```python
from build123d import *

# Parameters (mm, degrees)
BASE_FLANGE1_DEPTH                            = 43.6626
SKETCH3_W                                     = 39.3553177
SKETCH3_H                                     = 59.329005091
CUT_EXTRUDE1_DEPTH                            = 221.446361168
CSK_FOR_8_FLAT_HEAD_MACHINE_SCREW1_AT_2_COUNT = 2
CSK_FOR_8_FLAT_HEAD_MACHINE_SCREW1_AT_2_PITCH = 34.9504
SKETCH6_R                                     = 3.175
SKETCH6_R_2                                   = 2.0193
SKETCH6_R_3                                   = 2.7051
CUT_EXTRUDE2_DEPTH                            = 7.62
CUT_EXTRUDE3_REACH                            = 258.55
SKETCH7_R                                     = 2.7051
CE_00_NOTCH_FOR_WIRE_REACH                    = 222.446


# Sheet-metal steps are written as plain solids
with BuildPart() as part:
    # Sketch1 → Base-Flange1 (new, symmetric)
    with BuildSketch(Plane.XY):
        with BuildLine():
            Line((139.7, -25.4), (139.7, -40.559570335))
            ThreePointArc((139.7, -40.559570335), (139.568524729, -41.220541159), (139.194114832, -41.780885168))
            Line((139.194114832, -41.780885168), (-50.802114832, -231.777114832))
            ThreePointArc((-50.802114832, -231.777114832), (-51.362458841, -232.151524729), (-52.023429665, -232.283))
            Line((-52.023429665, -232.283), (-70.358, -232.283))
            Line((-70.358, -232.283), (-70.358, -234.569))
            Line((-70.358, -234.569), (-52.023429665, -234.569))
            ThreePointArc((-52.023429665, -234.569), (-50.487644514, -234.26351334), (-49.185668731, -233.393560934))
            Line((-49.185668731, -233.393560934), (140.810560934, -43.397331269))
            ThreePointArc((140.810560934, -43.397331269), (141.68051334, -42.095355486), (141.986, -40.559570335))
            Line((141.986, -40.559570335), (141.986, -25.4))
            Line((141.986, -25.4), (139.7, -25.4))
        make_face()
    extrude(amount=BASE_FLANGE1_DEPTH, both=True)

    # Sketch3 → Cut-Extrude1 (cut, through all)
    with BuildSketch(Plane(origin=(92.103946102, -92.103946102, 0), x_dir=(0, 0, -1), z_dir=(0.7071067811865464, -0.7071067811865487, 0))):
        with Locations((-56.20285885, -229.689502546)):
            Rectangle(SKETCH3_W, SKETCH3_H)
        with Locations((56.20285885, -229.689502546)):
            Rectangle(SKETCH3_W, SKETCH3_H)
    extrude(amount=-CUT_EXTRUDE1_DEPTH, mode=Mode.SUBTRACT)

    # Sketch4 → CSK for #8 Flat Head Machine Screw1 (revolve, cut)
    with BuildSketch(Plane(origin=(141.986, -33.3502, -17.4752), x_dir=(0, 0, -1), z_dir=(0, 1, 0))):
        Polygon((0, 0), (0, 2.286), (2.7051, 2.286), (2.7051, 1.738551774), (4.2164, 0), align=None)
    csk_for_8_flat_head_machine_screw1 = revolve(axis=Axis((148.336, -33.3502, -17.4752), (-1, 0, 0)), mode=Mode.SUBTRACT)

    # CSK for #8 Flat Head Machine Screw1 at 2: CSK for #8 Flat Head Machine Screw1 ×2
    with Locations(*[(0, 0, i * CSK_FOR_8_FLAT_HEAD_MACHINE_SCREW1_AT_2_PITCH) for i in range(1, CSK_FOR_8_FLAT_HEAD_MACHINE_SCREW1_AT_2_COUNT)]):
        add(csk_for_8_flat_head_machine_screw1, mode=Mode.SUBTRACT)

    # Sketch6 → Cut-Extrude2 (cut)
    with BuildSketch(Plane(origin=(92.103946102, -92.103946102, 0), x_dir=(0, 0, -1), z_dir=(0.7071067811865465, -0.7071067811865486, 0))):
        with Locations(Location((0, 56.896984938, 0), (0, 0, 90))):
            Circle(SKETCH6_R)
        with Locations(Location((25.4, 44.196984938, 0), (0, 0, 90))):
            Circle(SKETCH6_R_2)
        with Locations(Location((25.4, -32.003015062, 0), (0, 0, 90))):
            Circle(SKETCH6_R_2)
        with Locations(Location((25.4, -108.203015062, 0), (0, 0, 90))):
            Circle(SKETCH6_R_2)
        with Locations(Location((-25.4, -108.203015062, 0), (0, 0, 90))):
            Circle(SKETCH6_R_2)
        with Locations(Location((-25.4, -32.003015062, 0), (0, 0, 90))):
            Circle(SKETCH6_R_2)
        with Locations(Location((-25.4, 44.196984938, 0), (0, 0, 90))):
            Circle(SKETCH6_R_2)
        with Locations(Location((0, -32.003015062, 0), (0, 0, 90))):
            Circle(SKETCH6_R_3)
        with Locations(Location((25.4, -184.403015062, 0), (0, 0, 90))):
            Circle(SKETCH6_R_2)
        with Locations(Location((-25.4, -184.403015062, 0), (0, 0, 90))):
            Circle(SKETCH6_R_2)
        with Locations(Location((0, -83.518444727, 0), (0, 0, 90))):
            Circle(SKETCH6_R_3)
    extrude(amount=-CUT_EXTRUDE2_DEPTH, mode=Mode.SUBTRACT)

    # Sketch7 → Cut-Extrude3 (cut, up to next)
    with BuildSketch(Plane.XZ.offset(234.569), mode=Mode.PRIVATE) as cut_extrude3_sk1:
        with Locations((-63.5, 25.4)):
            Circle(SKETCH7_R)
    cut_extrude3_tool1 = extrude(cut_extrude3_sk1.sketch, amount=-CUT_EXTRUDE3_REACH, mode=Mode.PRIVATE) & part.part
    # Sketch7 → Cut-Extrude3 (cut, up to next)
    with BuildSketch(Plane.XZ.offset(234.569), mode=Mode.PRIVATE) as cut_extrude3_sk2:
        with Locations((-63.5, -25.4)):
            Circle(SKETCH7_R)
    cut_extrude3_tool2 = extrude(cut_extrude3_sk2.sketch, amount=-CUT_EXTRUDE3_REACH, mode=Mode.PRIVATE) & part.part
    add(cut_extrude3_tool1.solids().sort_by_distance((-63.5, -234.569, 25.4))[0], mode=Mode.SUBTRACT)
    add(cut_extrude3_tool2.solids().sort_by_distance((-63.5, -234.569, -25.4))[0], mode=Mode.SUBTRACT)

    # Sketch8 → CE-00 Notch for Wire (cut, up to next)
    with BuildSketch(Plane(origin=(92.103946102, -92.103946102, 0), x_dir=(0, 0, -1), z_dir=(0.7071067811865465, -0.7071067811865486, 0)), mode=Mode.PRIVATE) as ce_00_notch_for_wire_sk1:
        with BuildLine():
            Line((64.632412862, -80.216444727), (35.7124, -80.216444727))
            ThreePointArc((35.7124, -80.216444727), (32.4104, -83.518444727), (35.7124, -86.820444727))
            Line((35.7124, -86.820444727), (64.632412862, -86.820444727))
            Line((64.632412862, -86.820444727), (64.632412862, -80.216444727))
        make_face()
    ce_00_notch_for_wire_tool1 = extrude(ce_00_notch_for_wire_sk1.sketch, amount=-CE_00_NOTCH_FOR_WIRE_REACH, mode=Mode.PRIVATE) & part.part
    add(ce_00_notch_for_wire_tool1.solids().sort_by_distance((33.047487, -151.160405, -48.867096))[0], mode=Mode.SUBTRACT)


solid = part.part
```
Geometry: final body of the model. Coordinates: model frame, mm. A direction names the side the tool comes from. Coordinates: 2 decimals unless noted, no trailing zeros. Order: outer loops, then holes, each group sorted by start corner. A loop starts at its lowest first (then second) coordinate and runs counter-clockwise, first axis right, second up. Notation, with made-up numbers: (74.25, 58) -> (80.25, 58) arc R24 ccw to (80.25, 86) -> close; hole circle Ø2 at (31, 19.25). An arc over 180 degrees is marked (long way). Write item = value, one per line.
(1) Pull-direction query (Y, two-part tool) for faces 1 (the cylindrical face through (139.98, -30.95, -18.72)), 2 (the flat face through (45.526, -135.449, 0.611)), 3 (the flat face through (-61, -234.569, 1)); classes: pulls with the +Y half, pulls with the -Y half, needs draft (parallel to the pull), parting line crosses it, or undercut.
Solved:
face_1 = undercut
face_2 = pulls with the +Y half
face_3 = pulls with the -Y half
(2) Cut plane C-C on y = -138.5. Return loops of the section in (x, z) (3 decimals), plus the area to 3 significant figures.
Solved:
outline = (42.475, -43.663) -> (45.708, -43.663) -> (45.708, 43.663) -> (42.475, 43.663) -> close
area = 282 mm²
(3) Cut plane D-D on x = 78.5. Return loops of the section in (y, z) (3 decimals).
Solved:
outline = (-105.708, -43.663) -> (-102.475, -43.663) -> (-102.475, 43.663) -> (-105.708, 43.663) -> close
(4) Line query: line 1 (Z direction, x = -63.5, y = -232.85); line 2 (X direction, y = -36.5, z = 10); line 3 (Y direction, x = 100.5, z = -23.5) (3 decimals). Output: solid intervals per line, ascending.
Solved:
line_1 = -36.53 to -28.11, -22.69 to 22.69, 28.11 to 36.53
line_2 = 139.7 to 141.99
line_3 = -83.708 to -80.475
(5) Pin query (flat end, axial travel): pin 1 Ø6 at (x, z) = (-63.5, 25.4) entering from +Y; pin 2 Ø4 at (y, z) = (-142, 17) entering from +X; pin 3 Ø5 at (y, z) = (-155, -21) entering from -X (3 decimals). Return the tip coordinate at first contact, or that it passes through.
Solved:
pin_1 = -232.28
pin_2 = 44.21
pin_3 = 23.475
(6) Access query for faces 4 (the flat face through (96, -87, -43.663)), 5 (the flat face through (-61, -232.283, 1)). Directions: +Z, -Z, +X, -X, +Y, -Y. A direction counts if a zero-diameter tool reaches every point of the face in a straight line with its end or side. Return the directions, or none.
Solved:
face_4 = -Z, +X, -X, +Y, -Y
face_5 = +Z, -Z, -X, +Y
(7) Cut plane A-A on x = -63.5. Return loops of the section in (y, z).
Solved:
outline = (-234.57, -36.53) -> (-232.28, -36.53) -> (-232.28, -28.11) -> (-234.57, -28.11) -> close; (-234.57, -22.69) -> (-232.28, -22.69) -> (-232.28, 22.69) -> (-234.57, 22.69) -> close; (-234.57, 28.11) -> (-232.28, 28.11) -> (-232.28, 36.53) -> (-234.57, 36.53) -> close
(8) Cut plane B-B on z = 9. Return loops of the section in (x, y).
Solved:
outline = (-70.36, -234.57) -> (-52.02, -234.57) arc R4.01 ccw to (-49.19, -233.39) -> (140.81, -43.4) arc R4.01 ccw to (141.99, -40.56) -> (141.99, -25.4) -> (139.7, -25.4) -> (139.7, -40.56) arc R1.73 cw to (139.19, -41.78) -> (-50.8, -231.78) arc R1.73 cw to (-52.02, -232.28) -> (-70.36, -232.28) -> close
